For this review, take the finished solid that the model builds, in its own axes (mm). A direction names the side the tool comes from. Round coordinates to 2 decimals unless told otherwise and drop trailing zeros. Order: outer loops, then holes, each group sorted by start corner. A loop starts at its lowest first (then second) coordinate and runs counter-clockwise, first axis right, second up. Notation, with made-up numbers: (-9, -23) -> (49, -23) arc R24 cw to (49, -11) -> close; hole circle Ø7 at (-23.5, 50.5). An arc over 180 degrees is marked (long way). Use a Markdown table: item, result. Add a question column.
1) Draft analysis for pull direction Z (two halves, no side actions). For faces 1 (the face through (-8, 5, 0)), 2 (the face through (-5.06, 4, -7.62)), 3 (the face through (-6, 1.588, -11)), 4 (the face through (-12.798, 0.905, -15.758)), state which applies: pulls with the +Z half, pulls with the -Z half, needs draft (parallel to the pull), parting line crosses it, or undercut.
2) Machinability: for faces 5 (the face through (-3.91, 0.91, -0.95)), 6 (the face through (-0.91, 0.95, -12.89)), 7 (the face through (-15.808, 0.955, -3.826)), which of the approach directions +Z, -Z, +X, -X, +Y, -Y give a long, thin tool a straight path to every point of the face, cutting with its end or side? Answer none if there is none.
3) Wall thickness on line 1 along Y through (x, z) = (-9.75, -12.5); line 2 along X through (y, z) = (5.75, -6.5); line 3 along X through (y, z) = (4.25, -9.5): over which ranges is each line inside the solid? List them lowest first. Write a range as [from, to].
4) Consider section B-B (y = 5). State the section outline as (x, z) points, plus the area to 3 significant figures.
5) Clearance check with a flat-ended pin moving along its axis: P1, Ø5.5, axis at x = -7.5, z = -8.5, coming from the -Y side. State where the tip first meets the part, or that it passes through.
Autodesk Inventor part; units mm, degrees
ref_plane "YZ Plane" through (0, 0, 0) normal (1, 0, 0) x (0, 1, 0)
ref_plane "XZ Plane" through (0, 0, 0) normal (0, 1, 0) x (-1, 0, 0)
ref_plane "XY Plane" through (0, 0, 0) normal (0, 0, 1) x (1, 0, 0)
sketch "Sketch1" plane through (0, 0, 0) normal (0, 1, 0) x (-1, 0, 0)
  line L0 (0, 0) -> (16.7132, 0)
  line L1 (16.7132, 0) -> (16.7132, -16.7132)
  line L2 (16.7132, -16.7132) -> (0, -16.7132)
  line L3 (0, -16.7132) -> (0, 0)
  line L4 (16.7132, 0) -> (16.7132, -8.3566)
  line L5 (16.7132, -16.7132) -> (8.2065, -16.7132)
  line L6 (0, 0) -> (0, -8.3566)
  line L7 (0, -8.3566) -> (16.7132, -8.3566)
  line L8 (16.7132, -8.3566) -> (8.3566, -8.3566)
  dimension "d0" = 16.7132
  dimension "d1" = 16.7132
extrude "Extrusion1" add sketch "Sketch1" along normal blind 6.35
hole "Hole1" at (-8.3566, 0, -8.3566) direction (0, 1, 0) diameter 6.7564 end through all counterbore diameter 11.1252 counterbore depth 1.5875
fillet "Fillet1" radius 3.175 4 edges at (-8.3566, 0, 0) (-16.7132, 0, -8.3566) (0, 0, -8.3566) (-8.3566, 0, -16.7132)
properties part number "SquareRetainingClip"
Results list:
| question | item | result |
|---|---|---|
| 1 | face 1 | pulls with the +Z half |
| 1 | face 2 | undercut |
| 1 | face 3 | undercut |
| 1 | face 4 | pulls with the -Z half |
| 2 | face 5 | +Z, +X, -Y |
| 2 | face 6 | -Z, +X, -Y |
| 2 | face 7 | +Z, -X, -Y |
| 3 | line 1 | [1.59, 6.35] |
| 3 | line 2 | [-16.71, -11.18], [-5.53, 0] |
| 3 | line 3 | [-16.71, -11.54], [-5.18, 0] |
| 4 | outline | (-16.71, -16.71) -> (0, -16.71) -> (0, 0) -> (-16.71, 0) -> close; hole circle Ø6.76 at (-8.36, -8.36) |
| 4 | area | 243 mm2 |
| 5 | P1 | y = 1.59 |
